The listing builds one solid part. Answer for the finished solid, in the listing's coordinates (mm). Give positions to 0.01 mm unless a question says otherwise; leave off trailing zeros. Order: outer loops, then holes, each group sorted by start corner. A loop starts at its lowest first (then second) coordinate and runs counter-clockwise, first axis right, second up. Notation, with made-up numbers: (52, 25) - (67, 25) arc R32 ccw to (67, 53) - close; hole circle Ø11 at (-19, 65.25). An arc over 180 degrees is marked (long way). Answer as a JSON object with one key per item and string values. Group by question number.
Q1. A cutting plane is placed at B-B, the plane y = 0.9. Give the vertices of the cut face in (x, z), and give its area (3 significant figures).
Q2. A cutting plane is placed at A-A, the plane x = -38. Give the vertices of the cut face in (y, z).
Q3. The mould has two halves that part along Z. Classify faces 1 (the face through (-57.484, 1.014, -44.765)), 2 (the face through (-54.15, 1.01, -6.16)), 3 (the face through (-22, 0, -64)), 4 (the face through (-38.698, 0.986, -29.915)): released by +Z, released by -Z, zero draft, split by the parting line, or undercut.
Q4. Given pin 1 (1 mm diameter, centred on x = 1, y = 0.5, fed in from -Z); pin 2 (1 mm diameter, centred on y = 1, z = -55.5, fed in from +X), each flat-ended and moving along its own axis, determine where each tip first touches the part or whether it passes through.
Q5. Consider line 1 (Z direction, x = -40, y = 1); line 2 (X direction, y = 0.95, z = -26.5); line 3 (Z direction, x = -44.5, y = 1.9). Determine where each line is inside the solid, lowest interval first.
Q6. A cutting plane is placed at C-C, the plane z = -36.5. Give the vertices of the cut face in (x, y), and give its area (3 significant figures).
Q7. A cutting plane is placed at D-D, the plane z = -102.5. Give the vertices of the cut face in (x, y).
Autodesk Inventor part; units mm, degrees
ref_plane "YZ Plane" through (0, 0, 0) normal (1, 0, 0) x (0, 1, 0)
ref_plane "XZ Plane" through (0, 0, 0) normal (0, 1, 0) x (-1, 0, 0)
ref_plane "XY Plane" through (0, 0, 0) normal (0, 0, 1) x (1, 0, 0)
sketch "Sketch1" plane through (0, 0, 0) normal (0, 1, 0) x (-1, 0, 0)
  line L0 (0, 0) -> (60, 0)
  line L1 (60, 0) -> (60, -45)
  line L2 (60, -45) -> (20.3638, -130)
  line L3 (20.3638, -130) -> (0, -130)
  line L4 (0, 0) -> (0, -130)
  circle A0 centre (40, -20) radius 10
  line L5 (0, -20) -> (-2, -20)
  line L6 (-2, -20) -> (-2, -40)
  line L7 (-2, -40) -> (0, -40)
  line L8 (0, -40) -> (0, -20)
  line L9 (0, -90) -> (-2, -90)
  line L10 (-2, -90) -> (-2, -110)
  line L11 (-2, -110) -> (0, -110)
  line L12 (0, -110) -> (0, -90)
  dimension "d0" = 45
  dimension "d1" = 40
  dimension "d2" = 20
  dimension "d3" = 20
  dimension "d4" = 130
  dimension "d5" = 20
  dimension "d10" = 25
  dimension "d11" = 2
  dimension "d12" = 2
  dimension "d13" = 20
  dimension "d14" = 20
  dimension "d15" = 20
  dimension "d16" = 20
extrude "Plate1" add sketch "Sketch1" along normal blind 2
fillet "Fillet1" radius 20.5 1 edges at (-60, 1, 0)
fillet "Fillet2" radius 103.25 1 edges at (-60, 1, -45)
fillet "Fillet3" radius 15.5 1 edges at (-20.3638, 1, -130)
equation "\"d6\" = Thickness"
equation "\"BendRadius\" = Thickness"
equation "\"BendReliefWidth\" = Thickness"
equation "\"BendReliefDepth\" = 0.5 * Thickness"
equation "\"CornerReliefSize\" = 4 * Thickness"
equation "\"MinimumRemnant\" = 2 * Thickness"
equation "\"TransitionRadius\" = BendRadius"
equation "\"JacobiRadiusSize\" = BendRadius"
equation "\"GapSize\" = Thickness"
properties part number "Beslag_stempel"
Reply:
{
 "1": {"outline": "(-60, -22.11) arc R103.25 ccw to (-50.33, -65.75) - (-24.54, -121.05) arc R15.5 ccw to (-10.49, -130) - (0, -130) - (0, -110) - (2, -110) - (2, -90) - (0, -90) - (0, -40) - (2, -40) - (2, -20) - (0, -20) - (0, 0) - (-39.5, 0) arc R20.5 ccw to (-60, -20.5) - close; hole circle Ø20 at (-40, -20)", "area": "5,740 mm^2"},
 "2": {"outline": "(0, -92.18) - (2, -92.18) - (2, -29.8) - (0, -29.8) - close; (0, -10.2) - (2, -10.2) - (2, 0) - (0, 0) - close"},
 "3": {"face 1": "released by -Z", "face 2": "released by +Z", "face 3": "zero draft", "face 4": "undercut"},
 "4": {"pin 1": "stops at z = -110", "pin 2": "stops at x = 0"},
 "5": {"line 1": "z = -87.89 to -30, -10 to -0.01", "line 2": "x = -59.91 to -47.6, -32.4 to 2", "line 3": "z = -78.24 to -28.93, -11.07 to -0.62"},
 "6": {"outline": "(-58.99, 0) - (2, 0) - (2, 2) - (-58.99, 2) - close", "area": "122 mm^2"},
 "7": {"outline": "(-33.19, 0) - (2, 0) - (2, 2) - (-33.19, 2) - close"}
}
